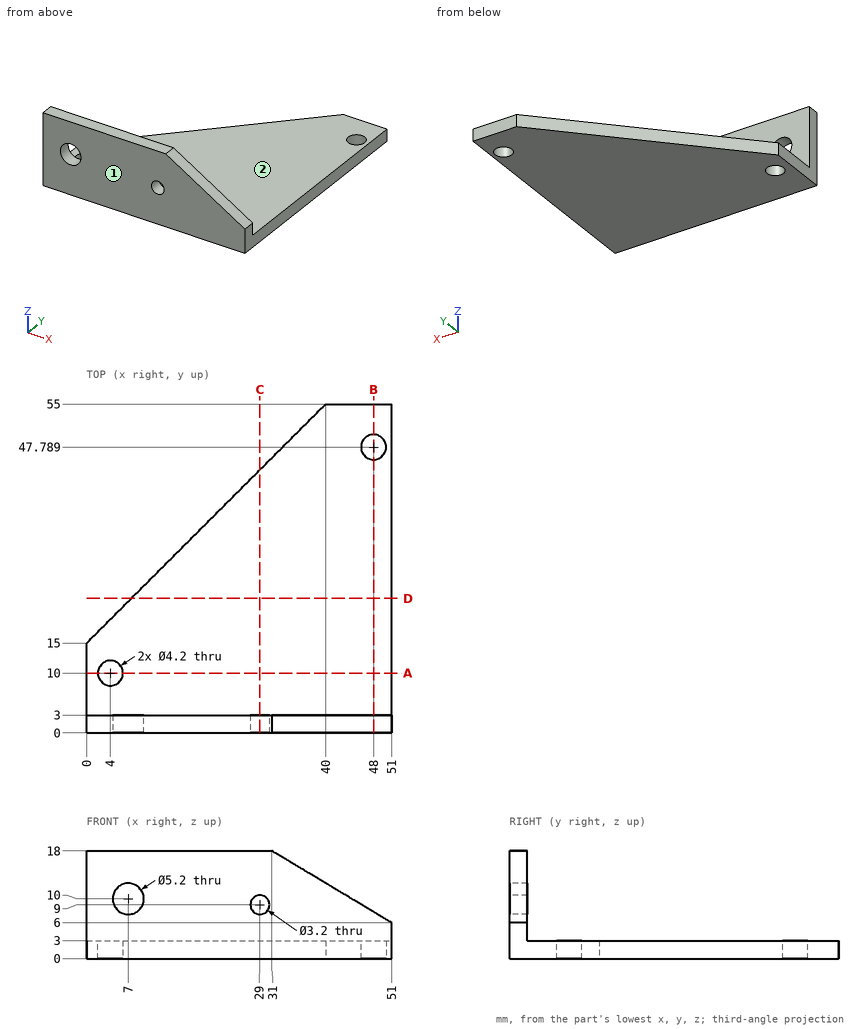
Drawing for the job (mm, zero at the part's lowest x, y, z). A direction names the side the tool comes from. Round coordinates to 2 decimals unless told otherwise and drop trailing zeros. Write each loop counter-clockwise with the first axis right and the second up, starting at its lowest first coordinate (ties: lowest second). Pieces come first, ordered by that corner, then holes. Notation, with made-up numbers: M 50.5,23 L 56.5,23 A23 ccw 56.5,54 Z; hole C 71,-13.5 d8. An arc over 180 degrees is marked long. Put each result on its own line as item: value.
Item 1: Cut at A-A (y = 10). List the corners of the cut face in (x, z).
Responses:
outline: M 0,0 L 1.9,0 L 1.9,3 L 0,3 Z; M 6.1,0 L 51,0 L 51,3 L 6.1,3 Z
Item 2: Probe L1, parallel to Y at x = 48, z = 1.05; L2, parallel to Y at x = 13, z = 3.75. List the from-to ranges inside material, lowest first. Write a range as from..to.
Responses:
L1: 0..45.69, 49.89..55
L2: 0..3
Item 3: Cut at B-B (x = 48). List the corners of the cut face in (y, z), and give its area (3 significant figures).
Responses:
outline: M 0,0 L 45.69,0 L 45.69,3 L 3,3 L 3,7.8 L 0,7.8 Z; M 49.89,0 L 55,0 L 55,3 L 49.89,3 Z
area: 167 mm²
Item 4: Flat gauge pins, fed straight in: P1, Ø15.5, axis at x = 29.5, y = 24.5, coming from the +Z side; P2, Ø4, axis at x = 21, z = 8, coming from the +Y side. Where does each tip first touch, or does it go through?
Responses:
P1: z = 3
P2: y = 3
Item 5: Cut at C-C (x = 29). List the corners of the cut face in (y, z).
Responses:
outline: M 0,0 L 44,0 L 44,3 L 3,3 L 3,7.4 L 0,7.4 Z; M 0,10.6 L 3,10.6 L 3,18 L 0,18 Z
Item 6: Tool access for the marked faces 1 and 2: list every direction of +Z, -Z, +X, -X, +Y, -Y with a clear straight run to the whole face (end or side of a thin tool).
Responses:
face 1: +Z, -Z, +X, -X, -Y
face 2: +Z, +X, -X, +Y
Item 7: Cut at D-D (y = 22.5). List the corners of the cut face in (x, z).
Responses:
outline: M 7.5,0 L 51,0 L 51,3 L 7.5,3 Z
